from build123d import *

# Parameters (mm, degrees)
SKETCH1_W           = 206
SKETCH1_H           = 81
SKETCH1_R           = 2
SKETCH1_R_2         = 11
SKETCH1_W_2         = 5
SKETCH1_H_2         = 5
BOSS_EXTRUDE1_DEPTH = 5
FILLET1_R           = 5
CUT_EXTRUDE1_DEPTH  = 0.5


with BuildPart() as part:
    # Sketch1 → Boss-Extrude1 (new body)
    with BuildSketch(Plane(origin=(0, 0, 0), x_dir=(1, 0, 0), z_dir=(0, 1, 0))):
        with Locations((5.102707087, 13.156325227)):
            Rectangle(SKETCH1_W, SKETCH1_H)
        with Locations(Location((-54.897292913, 48.156325227, 0), (0, 0, 270))):
            Circle(SKETCH1_R, mode=Mode.SUBTRACT)
        with Locations(Location((-54.897292913, -21.843674773, 0), (0, 0, 90))):
            Circle(SKETCH1_R, mode=Mode.SUBTRACT)
        with Locations(Location((65.102707087, -21.843674773, 0), (0, 0, 270))):
            Circle(SKETCH1_R, mode=Mode.SUBTRACT)
        with Locations(Location((65.102707087, 48.156325227, 0), (0, 0, 90))):
            Circle(SKETCH1_R, mode=Mode.SUBTRACT)
        with Locations(Location((-48.397292913, 13.156325227, 0), (0, 0, 270))):
            Circle(SKETCH1_R, mode=Mode.SUBTRACT)
        with Locations(Location((58.602707087, 13.156325227, 0), (0, 0, 90))):
            Circle(SKETCH1_R, mode=Mode.SUBTRACT)
        with Locations(Location((-74.397292913, 13.156325227, 0), (0, 0, 270))):
            Circle(SKETCH1_R_2, mode=Mode.SUBTRACT)
        with Locations((57.602707087, 48.156325227)):
            Rectangle(SKETCH1_W_2, SKETCH1_H_2, mode=Mode.SUBTRACT)
        with Locations((-62.397292913, 48.156325227)):
            Rectangle(SKETCH1_W_2, SKETCH1_H_2, mode=Mode.SUBTRACT)
        with Locations((-47.397292913, 48.156325227)):
            Rectangle(SKETCH1_W_2, SKETCH1_H_2, mode=Mode.SUBTRACT)
        with Locations((72.602707087, 48.156325227)):
            Rectangle(SKETCH1_W_2, SKETCH1_H_2, mode=Mode.SUBTRACT)
        with Locations((72.602707087, -21.843674773)):
            Rectangle(SKETCH1_W_2, SKETCH1_H_2, mode=Mode.SUBTRACT)
        with Locations((57.602707087, -21.843674773)):
            Rectangle(SKETCH1_W_2, SKETCH1_H_2, mode=Mode.SUBTRACT)
        with Locations((-47.397292913, -21.843674773)):
            Rectangle(SKETCH1_W_2, SKETCH1_H_2, mode=Mode.SUBTRACT)
        with Locations((-62.397292913, -21.843674773)):
            Rectangle(SKETCH1_W_2, SKETCH1_H_2, mode=Mode.SUBTRACT)
        with Locations((-48.397292913, 20.656325227)):
            Rectangle(SKETCH1_W_2, SKETCH1_H_2, mode=Mode.SUBTRACT)
        with Locations((-48.397292913, 5.656325227)):
            Rectangle(SKETCH1_W_2, SKETCH1_H_2, mode=Mode.SUBTRACT)
        with Locations((58.602707087, 5.656325227)):
            Rectangle(SKETCH1_W_2, SKETCH1_H_2, mode=Mode.SUBTRACT)
        with Locations((58.602707087, 20.656325227)):
            Rectangle(SKETCH1_W_2, SKETCH1_H_2, mode=Mode.SUBTRACT)
    extrude(amount=BOSS_EXTRUDE1_DEPTH)

    # Fillet1
    fillet1_edges = [part.edges().sort_by_distance(p)[0] for p in [
        (-97.897292913, 2.5, -53.656325227),
        (108.102707087, 2.5, -53.656325227),
        (108.102707087, 2.5, 27.343674773),
        (-97.897292913, 2.5, 27.343674773),
    ]]
    fillet(fillet1_edges, radius=FILLET1_R)

    # Sketch2 → Cut-Extrude1 (cut)
    with BuildSketch(Plane(origin=(0, 5, 0), x_dir=(1, 0, 0), z_dir=(0, 1, 0))):
        Polygon((-39.897292913, 18.396325227), (-39.897292913, -14.003674773), (5.102707087, -14.003674773), (5.102707087, -10.943674773), (-36.837292913, -10.943674773), (-36.837292913, 17.128831726), (-16.714799412, 37.251325227), (5.102707087, 37.251325227), (5.102707087, 40.311325227), (-17.982292913, 40.311325227), align=None)
        Polygon((5.102707087, -10.943674773), (5.102707087, -14.003674773), (50.102707087, -14.003674773), (50.102707087, 18.396325227), (28.187707087, 40.311325227), (5.102707087, 40.311325227), (5.102707087, 37.251325227), (26.920213586, 37.251325227), (47.042707087, 17.128831726), (47.042707087, -10.943674773), align=None)
        Polygon((5.102707087, -4.013674773), (5.102707087, -7.883674773), (43.982707087, -7.883674773), (43.982707087, 15.861338225), (25.652720085, 34.191325227), (5.102707087, 34.191325227), (5.102707087, 28.791325227), (21.302707087, 28.791325227), (21.302707087, 15.741325227), (12.842707087, 15.741325227), (12.842707087, -4.013674773), align=None)
        Polygon((-33.777292913, -7.883674773), (5.102707087, -7.883674773), (5.102707087, -4.013674773), (-2.637292913, -4.013674773), (-2.637292913, 15.741325227), (-11.097292913, 15.741325227), (-11.097292913, 28.791325227), (5.102707087, 28.791325227), (5.102707087, 34.191325227), (-15.447305912, 34.191325227), (-33.777292913, 15.861338225), align=None)
        Polygon((0.422707087, -0.953674773), (5.102707087, -0.953674773), (5.102707087, 25.731325227), (-8.037292913, 25.731325227), (-8.037292913, 18.801325227), (0.422707087, 18.801325227), align=None)
        Polygon((5.102707087, 25.731325227), (5.102707087, -0.953674773), (9.782707087, -0.953674773), (9.782707087, 18.801325227), (18.242707087, 18.801325227), (18.242707087, 25.731325227), align=None)
    extrude(amount=-CUT_EXTRUDE1_DEPTH, mode=Mode.SUBTRACT)


solid = part.part
Check sheet for the modelled part. Datum: model origin and axes. Units: mm. A direction names the side the tool comes from. Round coordinates to 2 decimals unless told otherwise and drop trailing zeros. Loops run counter-clockwise (first coordinate to the right, second up) from the corner with the lowest first, then second, coordinate; pieces in that order, holes last.
1. Mould release check, pull along X, two halves, no side actions. Record for faces 1 (the cylindrical face through (65.869, 2.465, -50.004)), 2 (the flat face through (4, 2, 27.344)): released by +X, released by -X, zero draft, split by the parting line, or undercut.
2. Sectioned sample at A-A on x = -22. Record the boundary of the cut face in (y, z).
3. Sectioned sample at B-B on y = 3.15. Give the number of separate pieces and of enclosed holes in the cut face, and give its area (3 significant figures).
4. Set-up check for faces 3 (the flat face through (-28.786, 4.754, -29.507)), 4 (the flat face through (-59.897, 2, 22)): record each of +Z, -Z, +X, -X, +Y, -Y from which the full face is reachable in a straight line by a thin tool's end or side.
5. Gauge pin test, flat end, axial feed: pin 1 Ø17.5 at (x, z) = (-74.4, -13.16) entering from -Y. Record the tip position at first contact, or that the pin passes through.
6. Scan lines: probe 1 along Z at (x, y) = (-55.5, 3.65); probe 2 along X at (y, z) = (3.85, -12.5); probe 3 along X at (y, z) = (0.6, -21.5). Record each from-to range of solid material in increasing order.
7. Sectioned sample at C-C on x = 36. Record the boundary of the cut face in (y, z), and give its area (3 significant figures).
Recorded:
1. face 1: undercut
1. face 2: zero draft
2. outline: (0, -53.66) - (5, -53.66) - (5, -36.29) - (4.5, -36.29) - (4.5, -31.97) - (5, -31.97) - (5, -27.64) - (4.5, -27.64) - (4.5, 7.88) - (5, 7.88) - (5, 10.94) - (4.5, 10.94) - (4.5, 14) - (5, 14) - (5, 27.34) - (0, 27.34) - close
3. separate pieces: 1
3. enclosed holes: 19
3. area: 15,900 mm2
4. face 3: +Y
4. face 4: +Y, -Y
5. pin 1: passes through
6. probe 1: z = -53.66 to -50.06, -46.25 to 19.94, 23.75 to 27.34
6. probe 2: x = -97.9 to -85.38, -63.42 to -50.29, -46.51 to 56.71, 60.49 to 108.1
6. probe 3: x = -97.9 to -81.57, -67.23 to -50.9, -45.9 to 56.1, 61.1 to 108.1
7. outline: (0, -53.66) - (5, -53.66) - (5, -32.5) - (4.5, -32.5) - (4.5, -28.17) - (5, -28.17) - (5, -23.84) - (4.5, -23.84) - (4.5, 7.88) - (5, 7.88) - (5, 10.94) - (4.5, 10.94) - (4.5, 14) - (5, 14) - (5, 27.34) - (0, 27.34) - close
7. area: 385 mm2
